For this review, take the finished solid that the model builds, in its own axes (mm). Face numbers are marked on the shaded views. A direction names the side the tool comes from. Round coordinates to 2 decimals unless told otherwise and drop trailing zeros. Write each loop counter-clockwise with the first axis right and the second up, starting at its lowest first coordinate (ties: lowest second). Pieces come first, ordered by that corner, then holes. Notation, with made-up numbers: (78, 44) - (124, 44) arc R21 cw to (124, 82) - close; hole circle Ø6 at (-3.5, -7.75). An arc over 180 degrees is marked (long way). One line per item, written item: value. Start each with the question number.
Q1. Add section C-C on z = 13. Write out the cut boundary in (x, y), and give its area (3 significant figures).
Q2. Clearance check with flat-ended pins moving along their axes: pin 1 Ø15.5 at (y, z) = (41.5, 26.5) entering from -X; pin 2 Ø5.5 at (x, y) = (-36.93, 15.46) entering from -Z; pin 3 Ø12 at (x, z) = (-19, 19) entering from +Y. State where each tip first meets the part, or that it passes through.
Q3. Add section B-B on y = 41.5. Write out the cut boundary in (x, z), and give its area (3 significant figures).
Q4. For probe 1 along Y at (x, z) = (-7, 26); probe 2 along X at (y, z) = (27, 8.5); probe 3 along X at (y, z) = (24.5, 16), list the stretches that pass through material, from the lowest coordinate up.
Q5. Add section A-A on x = -27. Write out the cut boundary in (y, z).
Q6. Tool access review of the marked faces 1, 2 and 3: name each direction out of +Z, -Z, +X, -X, +Y, -Y from which nothing blocks a thin tool from reaching the whole face with its end or side.
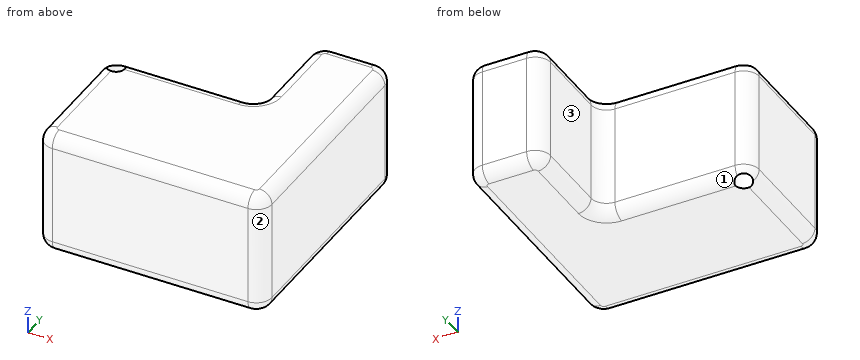
```python
from build123d import *

# Parameters (mm, degrees)
F0_R         = 3.3955807327
F1_DEPTH     = 50.8
F2_T1_DEPTH  = 79.7933701754
F2_T3_DEPTH  = 85.3559065938
F2_T5_DEPTH  = 18.0880006731
F2_T7_DEPTH  = 30.5066917419
F2_T9_DEPTH  = 49.0053695023
F2_T11_DEPTH = 42.1492148519
F2_T14_ANGLE = 90
F2_T16_ANGLE = 90
F2_T18_ANGLE = 90
F2_T20_ANGLE = 90
F2_T22_ANGLE = 90
F2_T24_ANGLE = 90
F2_T26_ANGLE = 90
F2_T28_ANGLE = 90
F2_T30_ANGLE = 90
F2_T32_ANGLE = 90
F2_T34_ANGLE = 90
F2_T36_ANGLE = 90


# Not quite as in the source:
# - a fillet or chamfer that OpenCascade refuses, or shapes differently, is made with other operations: its cross-section is extruded or revolved along the edge and cut away or added


with BuildPart() as f1:
    # F0 (on Top) → F1 (new body)
    with BuildSketch(Plane.XY):
        with BuildLine():
            Line((12.9895242095, 20.2450528741), (-36.0158452928, 20.2450528741))
            ThreePointArc((-36.0158452928, 20.2450528741), (-40.5059733533, 18.3851809346), (-42.3658452928, 13.8950528741))
            Line((-42.3658452928, 13.8950528741), (-42.3658452928, -28.2541619778))
            ThreePointArc((-42.3658452928, -28.2541619778), (-40.5059733533, -32.7442900383), (-36.0158452928, -34.6041619778))
            Line((-36.0158452928, -34.6041619778), (43.7775248826, -34.6041619778))
            ThreePointArc((43.7775248826, -34.6041619778), (48.2676529431, -32.7442900383), (50.1275248826, -28.2541619778))
            Line((50.1275248826, -28.2541619778), (50.1275248826, 20.2450528741))
            Line((50.1275248826, 20.2450528741), (50.1275248826, 57.101744616))
            ThreePointArc((50.1275248826, 57.101744616), (48.2676529431, 61.5918726766), (43.7775248826, 63.451744616))
            Line((43.7775248826, 63.451744616), (25.6895242095, 63.451744616))
            ThreePointArc((25.6895242095, 63.451744616), (21.199396149, 61.5918726766), (19.3395242095, 57.101744616))
            Line((19.3395242095, 57.101744616), (19.3395242095, 26.5950528741))
            ThreePointArc((19.3395242095, 26.5950528741), (17.47965227, 22.1049248136), (12.9895242095, 20.2450528741))
        make_face()
        with Locations((-36.93266958, 15.458682552)):
            Circle(F0_R, mode=Mode.SUBTRACT)
    extrude(amount=F1_DEPTH)

    # F2: fillet of radius 5.08 on 2 edges, made by hand

    # F2_s2 → F2_t1 (cut)
    with BuildSketch(Plane.YZ.offset(-36.0158452928)):
        with BuildLine():
            ThreePointArc((-29.5241619778, 50.8), (-33.1162644262, 49.3121024484), (-34.6041619778, 45.72))
            Line((-34.6041619778, 45.72), (-34.6041619778, 50.8))
            Line((-34.6041619778, 50.8), (-29.5241619778, 50.8))
        make_face()
        with BuildLine():
            ThreePointArc((-34.6041619778, 5.08), (-33.1162644262, 1.4878975516), (-29.5241619778, 0))
            Line((-29.5241619778, 0), (-34.6041619778, 0))
            Line((-34.6041619778, 0), (-34.6041619778, 5.08))
        make_face()
    extrude(amount=F2_T1_DEPTH, mode=Mode.SUBTRACT)

    # F2_s4 → F2_t3 (cut)
    with BuildSketch(Plane.XZ.offset(-57.101744616)):
        with BuildLine():
            ThreePointArc((50.1275248826, 5.08), (48.639627331, 1.4878975516), (45.0475248826, 0))
            Line((45.0475248826, 0), (50.1275248826, 0))
            Line((50.1275248826, 0), (50.1275248826, 5.08))
        make_face()
        with BuildLine():
            ThreePointArc((45.0475248826, 50.8), (48.639627331, 49.3121024484), (50.1275248826, 45.72))
            Line((50.1275248826, 45.72), (50.1275248826, 50.8))
            Line((50.1275248826, 50.8), (45.0475248826, 50.8))
        make_face()
    extrude(amount=F2_T3_DEPTH, mode=Mode.SUBTRACT)

    # F2_s6 → F2_t5 (cut)
    with BuildSketch(Plane.YZ.offset(25.6895242095)):
        with BuildLine():
            ThreePointArc((63.451744616, 5.08), (61.9638470645, 1.4878975516), (58.371744616, 0))
            Line((58.371744616, 0), (63.451744616, 0))
            Line((63.451744616, 0), (63.451744616, 5.08))
        make_face()
        with BuildLine():
            ThreePointArc((58.371744616, 50.8), (61.9638470645, 49.3121024484), (63.451744616, 45.72))
            Line((63.451744616, 45.72), (63.451744616, 50.8))
            Line((63.451744616, 50.8), (58.371744616, 50.8))
        make_face()
    extrude(amount=F2_T5_DEPTH, mode=Mode.SUBTRACT)

    # F2_s8 → F2_t7 (cut)
    with BuildSketch(Plane.XZ.offset(-57.101744616)):
        with BuildLine():
            ThreePointArc((24.4195242095, 0), (20.8274217611, 1.4878975516), (19.3395242095, 5.08))
            Line((19.3395242095, 5.08), (19.3395242095, 0))
            Line((19.3395242095, 0), (24.4195242095, 0))
        make_face()
        with BuildLine():
            ThreePointArc((24.4195242095, 50.8), (20.8274217611, 49.3121024484), (19.3395242095, 45.72))
            Line((19.3395242095, 45.72), (19.3395242095, 50.8))
            Line((19.3395242095, 50.8), (24.4195242095, 50.8))
        make_face()
    extrude(amount=F2_T7_DEPTH, mode=Mode.SUBTRACT)

    # F2_s10 → F2_t9 (cut)
    with BuildSketch(Plane.YZ.offset(-36.0158452928)):
        with BuildLine():
            ThreePointArc((15.1650528741, 0), (18.7571553225, 1.4878975516), (20.2450528741, 5.08))
            Line((20.2450528741, 5.08), (20.2450528741, 0))
            Line((20.2450528741, 0), (15.1650528741, 0))
        make_face()
        with BuildLine():
            ThreePointArc((15.1650528741, 50.8), (18.7571553225, 49.3121024484), (20.2450528741, 45.72))
            Line((20.2450528741, 45.72), (20.2450528741, 50.8))
            Line((20.2450528741, 50.8), (15.1650528741, 50.8))
        make_face()
    extrude(amount=F2_T9_DEPTH, mode=Mode.SUBTRACT)

    # F2_s12 → F2_t11 (cut)
    with BuildSketch(Plane.XZ.offset(-13.8950528741)):
        with BuildLine():
            ThreePointArc((-42.3658452928, 5.08), (-40.8779477412, 1.4878975516), (-37.2858452928, 0))
            Line((-37.2858452928, 0), (-42.3658452928, 0))
            Line((-42.3658452928, 0), (-42.3658452928, 5.08))
        make_face()
        with BuildLine():
            ThreePointArc((-37.2858452928, 50.8), (-40.8779477412, 49.3121024484), (-42.3658452928, 45.72))
            Line((-42.3658452928, 45.72), (-42.3658452928, 50.8))
            Line((-42.3658452928, 50.8), (-37.2858452928, 50.8))
        make_face()
    extrude(amount=F2_T11_DEPTH, mode=Mode.SUBTRACT)

    # F2_s13 → F2_t14 (revolve, cut)
    with BuildSketch(Plane.XZ.offset(28.2541619778)):
        with BuildLine():
            ThreePointArc((-42.3658452928, 5.08), (-40.8779477412, 1.4878975516), (-37.2858452928, 0))
            Line((-37.2858452928, 0), (-42.3658452928, 0))
            Line((-42.3658452928, 0), (-42.3658452928, 5.08))
        make_face()
    revolve(axis=Axis((-36.0158452928, -28.2541619778, 0), (0, 0, 1)), revolution_arc=F2_T14_ANGLE, mode=Mode.SUBTRACT)

    # F2_s15 → F2_t16 (revolve, cut)
    with BuildSketch(Plane.YZ.offset(43.7775248826)):
        with BuildLine():
            ThreePointArc((-34.6041619778, 5.08), (-33.1162644262, 1.4878975516), (-29.5241619778, 0))
            Line((-29.5241619778, 0), (-34.6041619778, 0))
            Line((-34.6041619778, 0), (-34.6041619778, 5.08))
        make_face()
    revolve(axis=Axis((43.7775248826, -28.2541619778, 0), (0, 0, 1)), revolution_arc=F2_T16_ANGLE, mode=Mode.SUBTRACT)

    # F2_s17 → F2_t18 (revolve, cut)
    with BuildSketch(Plane.XZ.offset(-57.101744616)):
        with BuildLine():
            ThreePointArc((50.1275248826, 5.08), (48.639627331, 1.4878975516), (45.0475248826, 0))
            Line((45.0475248826, 0), (50.1275248826, 0))
            Line((50.1275248826, 0), (50.1275248826, 5.08))
        make_face()
    revolve(axis=Axis((43.7775248826, 57.101744616, 0), (0, 0, 1)), revolution_arc=F2_T18_ANGLE, mode=Mode.SUBTRACT)

    # F2_s19 → F2_t20 (revolve, cut)
    with BuildSketch(Plane.YZ.offset(25.6895242095)):
        with BuildLine():
            ThreePointArc((63.451744616, 5.08), (61.9638470645, 1.4878975516), (58.371744616, 0))
            Line((58.371744616, 0), (63.451744616, 0))
            Line((63.451744616, 0), (63.451744616, 5.08))
        make_face()
    revolve(axis=Axis((25.6895242095, 57.101744616, 0), (0, 0, 1)), revolution_arc=F2_T20_ANGLE, mode=Mode.SUBTRACT)

    # F2_s21 → F2_t22 (revolve, cut)
    with BuildSketch(Plane.XZ.offset(-26.5950528741)):
        with BuildLine():
            ThreePointArc((19.3395242095, 5.08), (20.8274217611, 1.4878975516), (24.4195242095, 0))
            Line((24.4195242095, 0), (19.3395242095, 0))
            Line((19.3395242095, 0), (19.3395242095, 5.08))
        make_face()
    revolve(axis=Axis((12.9895242095, 26.5950528741, 0), (0, 0, -1)), revolution_arc=F2_T22_ANGLE, mode=Mode.SUBTRACT)

    # F2_s23 → F2_t24 (revolve, cut)
    with BuildSketch(Plane.YZ.offset(-36.0158452928)):
        with BuildLine():
            ThreePointArc((20.2450528741, 5.08), (18.7571553225, 1.4878975516), (15.1650528741, 0))
            Line((15.1650528741, 0), (20.2450528741, 0))
            Line((20.2450528741, 0), (20.2450528741, 5.08))
        make_face()
    revolve(axis=Axis((-36.0158452928, 13.8950528741, 0), (0, 0, 1)), revolution_arc=F2_T24_ANGLE, mode=Mode.SUBTRACT)

    # F2_s25 → F2_t26 (revolve, cut)
    with BuildSketch(Plane.XZ.offset(28.2541619778)):
        with BuildLine():
            ThreePointArc((-37.2858452928, 50.8), (-40.8779477412, 49.3121024484), (-42.3658452928, 45.72))
            Line((-42.3658452928, 45.72), (-42.3658452928, 50.8))
            Line((-42.3658452928, 50.8), (-37.2858452928, 50.8))
        make_face()
    revolve(axis=Axis((-36.0158452928, -28.2541619778, 50.8), (0, 0, 1)), revolution_arc=F2_T26_ANGLE, mode=Mode.SUBTRACT)

    # F2_s27 → F2_t28 (revolve, cut)
    with BuildSketch(Plane.YZ.offset(43.7775248826)):
        with BuildLine():
            ThreePointArc((-29.5241619778, 50.8), (-33.1162644262, 49.3121024484), (-34.6041619778, 45.72))
            Line((-34.6041619778, 45.72), (-34.6041619778, 50.8))
            Line((-34.6041619778, 50.8), (-29.5241619778, 50.8))
        make_face()
    revolve(axis=Axis((43.7775248826, -28.2541619778, 50.8), (0, 0, 1)), revolution_arc=F2_T28_ANGLE, mode=Mode.SUBTRACT)

    # F2_s29 → F2_t30 (revolve, cut)
    with BuildSketch(Plane.XZ.offset(-57.101744616)):
        with BuildLine():
            ThreePointArc((45.0475248826, 50.8), (48.639627331, 49.3121024484), (50.1275248826, 45.72))
            Line((50.1275248826, 45.72), (50.1275248826, 50.8))
            Line((50.1275248826, 50.8), (45.0475248826, 50.8))
        make_face()
    revolve(axis=Axis((43.7775248826, 57.101744616, 50.8), (0, 0, 1)), revolution_arc=F2_T30_ANGLE, mode=Mode.SUBTRACT)

    # F2_s31 → F2_t32 (revolve, cut)
    with BuildSketch(Plane.YZ.offset(25.6895242095)):
        with BuildLine():
            ThreePointArc((58.371744616, 50.8), (61.9638470645, 49.3121024484), (63.451744616, 45.72))
            Line((63.451744616, 45.72), (63.451744616, 50.8))
            Line((63.451744616, 50.8), (58.371744616, 50.8))
        make_face()
    revolve(axis=Axis((25.6895242095, 57.101744616, 50.8), (0, 0, 1)), revolution_arc=F2_T32_ANGLE, mode=Mode.SUBTRACT)

    # F2_s33 → F2_t34 (revolve, cut)
    with BuildSketch(Plane.XZ.offset(-26.5950528741)):
        with BuildLine():
            ThreePointArc((19.3395242095, 45.72), (20.8274217611, 49.3121024484), (24.4195242095, 50.8))
            Line((24.4195242095, 50.8), (19.3395242095, 50.8))
            Line((19.3395242095, 50.8), (19.3395242095, 45.72))
        make_face()
    revolve(axis=Axis((12.9895242095, 26.5950528741, 50.8), (0, 0, -1)), revolution_arc=F2_T34_ANGLE, mode=Mode.SUBTRACT)

    # F2_s35 → F2_t36 (revolve, cut)
    with BuildSketch(Plane.YZ.offset(-36.0158452928)):
        with BuildLine():
            ThreePointArc((15.1650528741, 50.8), (18.7571553225, 49.3121024484), (20.2450528741, 45.72))
            Line((20.2450528741, 45.72), (20.2450528741, 50.8))
            Line((20.2450528741, 50.8), (15.1650528741, 50.8))
        make_face()
    revolve(axis=Axis((-36.0158452928, 13.8950528741, 50.8), (0, 0, 1)), revolution_arc=F2_T36_ANGLE, mode=Mode.SUBTRACT)


solid = f1.part
```
Result set:
1. outline: (-42.37, -28.25) arc R6.35 ccw to (-36.02, -34.6) - (43.78, -34.6) arc R6.35 ccw to (50.13, -28.25) - (50.13, 57.1) arc R6.35 ccw to (43.78, 63.45) - (25.69, 63.45) arc R6.35 ccw to (19.34, 57.1) - (19.34, 26.6) arc R6.35 cw to (12.99, 20.25) - (-36.02, 20.25) arc R6.35 ccw to (-42.37, 13.9) - close; hole circle Ø6.79 at (-36.93, 15.46)
1. area: 6,330 mm^2
2. pin 1: stops at x = 19.34
2. pin 2: passes through
2. pin 3: stops at y = 20.25
3. outline: (19.34, 5.08) arc R5.08 ccw to (24.42, 0) - (45.05, 0) arc R5.08 ccw to (50.13, 5.08) - (50.13, 45.72) arc R5.08 ccw to (45.05, 50.8) - (24.42, 50.8) arc R5.08 ccw to (19.34, 45.72) - close
3. area: 1,540 mm^2
4. probe 1: y = -34.6 to 20.25
4. probe 2: x = 19.34 to 50.13
4. probe 3: x = 18.98 to 50.13
5. outline: (-34.6, 5.08) arc R5.08 ccw to (-29.52, 0) - (15.17, 0) arc R5.08 ccw to (20.25, 5.08) - (20.25, 45.72) arc R5.08 ccw to (15.17, 50.8) - (-29.52, 50.8) arc R5.08 ccw to (-34.6, 45.72) - close
6. face 1: -Z, -X, +Y
6. face 2: +Z, -Z, +X, -Y
6. face 3: +Z, -Z, -X, +Y
